```python
from build123d import *

# Parameters (mm, degrees)
SKETCH1_W           = 292.1
SKETCH1_H           = 158.75
BOSS_EXTRUDE1_DEPTH = 6.35
SKETCH2_R           = 3.175
CUT_EXTRUDE2_DEPTH  = 6.35
SKETCH4_R           = 2.54
SKETCH4_R_2         = 1.651
SKETCH4_R_3         = 2.667
SKETCH4_R_4         = 1.69999914
SKETCH4_R_5         = 2.0955
CUT_EXTRUDE5_DEPTH  = 333.512097524


with BuildPart() as part:
    # Sketch1 → Boss-Extrude1 (new body)
    with BuildSketch(Plane(origin=(0, 0, 0), x_dir=(1, 0, 0), z_dir=(0, 1, 0))):
        with Locations((146.05, 79.375)):
            Rectangle(SKETCH1_W, SKETCH1_H)
    extrude(amount=BOSS_EXTRUDE1_DEPTH)

    # Sketch2 → Cut-Extrude2 (cut)
    with BuildSketch(Plane(origin=(0, 6.35, 0), x_dir=(1, 0, 0), z_dir=(0, 1, 0))):
        with Locations(Location((146.05, 12.7, 0), (0, 0, 270))):
            Circle(SKETCH2_R)
        with Locations(Location((247.65, 12.7, 0), (0, 0, 270))):
            Circle(SKETCH2_R)
        with Locations(Location((44.45, 12.7, 0), (0, 0, 270))):
            Circle(SKETCH2_R)
    extrude(amount=-CUT_EXTRUDE2_DEPTH, mode=Mode.SUBTRACT)

    # Sketch4 → Cut-Extrude5 (cut, through all)
    with BuildSketch(Plane(origin=(0, 6.35, 0), x_dir=(1, 0, 0), z_dir=(0, 1, 0))):
        with Locations(Location((88.2015, 92.075, 0), (0, 0, 270))):
            Circle(SKETCH4_R)
        with Locations(Location((44.45, 111.125, 0), (0, 0, 270))):
            Circle(SKETCH4_R_2)
        with Locations(Location((44.45, 79.375, 0), (0, 0, 270))):
            Circle(SKETCH4_R_2)
        with Locations(Location((44.45, 47.625, 0), (0, 0, 270))):
            Circle(SKETCH4_R_2)
        with Locations(Location((10.795, 111.125, 0), (0, 0, 270))):
            Circle(SKETCH4_R_2)
        with Locations(Location((10.795, 79.375, 0), (0, 0, 270))):
            Circle(SKETCH4_R_2)
        with Locations(Location((10.795, 47.625, 0), (0, 0, 270))):
            Circle(SKETCH4_R_2)
        with Locations(Location((139.0015, 92.075, 0), (0, 0, 270))):
            Circle(SKETCH4_R)
        with Locations(Location((189.8015, 92.075, 0), (0, 0, 270))):
            Circle(SKETCH4_R)
        with Locations(Location((218.4146, 49.9364, 0), (0, 0, 270))):
            Circle(SKETCH4_R)
        with Locations(Location((285.0896, 49.9364, 0), (0, 0, 270))):
            Circle(SKETCH4_R)
        with Locations(Location((268.097, 139.3, 0), (0, 0, 270))):
            Circle(SKETCH4_R_3)
        with Locations(Location((268.097, 89.3, 0), (0, 0, 270))):
            Circle(SKETCH4_R_3)
        with Locations(Location((201.40419192, 147.125001204, 0), (0, 0, 270))):
            Circle(SKETCH4_R_4)
        with Locations(Location((157.90419256, 147.124999631, 0), (0, 0, 270))):
            Circle(SKETCH4_R_4)
        with Locations(Location((139.83529192, 147.125001204, 0), (0, 0, 270))):
            Circle(SKETCH4_R_4)
        with Locations(Location((96.33529256, 147.124999631, 0), (0, 0, 270))):
            Circle(SKETCH4_R_4)
        with Locations(Location((78.26639192, 147.125001204, 0), (0, 0, 270))):
            Circle(SKETCH4_R_4)
        with Locations(Location((34.76639256, 147.124999631, 0), (0, 0, 270))):
            Circle(SKETCH4_R_4)
        with Locations(Location((157.90419746, 11.624998851, 0), (0, 0, 270))):
            Circle(SKETCH4_R_4)
        with Locations(Location((201.40419682, 11.625000424, 0), (0, 0, 270))):
            Circle(SKETCH4_R_4)
        with Locations(Location((139.83529682, 11.625000424, 0), (0, 0, 270))):
            Circle(SKETCH4_R_4)
        with Locations(Location((96.33529746, 11.624998851, 0), (0, 0, 270))):
            Circle(SKETCH4_R_4)
        with Locations(Location((78.26639682, 11.625000424, 0), (0, 0, 270))):
            Circle(SKETCH4_R_4)
        with Locations(Location((34.76639746, 11.624998851, 0), (0, 0, 270))):
            Circle(SKETCH4_R_4)
        with Locations(Location((218.69969445, 141.2875, 0), (0, 0, 270))):
            Circle(SKETCH4_R_5)
        with BuildLine():
            Line((92.33531063, 130.175), (92.33531063, 120.65))
            ThreePointArc((92.33531063, 120.65), (89.16031063, 117.475), (85.98531063, 120.65))
            Line((85.98531063, 120.65), (85.98531063, 130.175))
            ThreePointArc((85.98531063, 130.175), (89.16031063, 133.35), (92.33531063, 130.175))
        make_face()
        with BuildLine():
            Line((30.76641063, 130.175), (30.76641063, 120.65))
            ThreePointArc((30.76641063, 120.65), (27.59141063, 117.475), (24.41641063, 120.65))
            Line((24.41641063, 120.65), (24.41641063, 130.175))
            ThreePointArc((24.41641063, 130.175), (27.59141063, 133.35), (30.76641063, 130.175))
        make_face()
        with BuildLine():
            Line((153.90421063, 130.175), (153.90421063, 120.65))
            ThreePointArc((153.90421063, 120.65), (150.72921063, 117.475), (147.55421063, 120.65))
            Line((147.55421063, 120.65), (147.55421063, 130.175))
            ThreePointArc((147.55421063, 130.175), (150.72921063, 133.35), (153.90421063, 130.175))
        make_face()
        with BuildLine():
            Line((153.90421063, 38.1), (153.90421063, 28.575))
            ThreePointArc((153.90421063, 28.575), (150.72921063, 25.4), (147.55421063, 28.575))
            Line((147.55421063, 28.575), (147.55421063, 38.1))
            ThreePointArc((147.55421063, 38.1), (150.72921063, 41.275), (153.90421063, 38.1))
        make_face()
        with BuildLine():
            Line((30.76641063, 38.1), (30.76641063, 28.575))
            ThreePointArc((30.76641063, 28.575), (27.59141063, 25.4), (24.41641063, 28.575))
            Line((24.41641063, 28.575), (24.41641063, 38.1))
            ThreePointArc((24.41641063, 38.1), (27.59141063, 41.275), (30.76641063, 38.1))
        make_face()
        with BuildLine():
            Line((92.33531063, 38.1), (92.33531063, 28.575))
            ThreePointArc((92.33531063, 28.575), (89.16031063, 25.4), (85.98531063, 28.575))
            Line((85.98531063, 28.575), (85.98531063, 38.1))
            ThreePointArc((85.98531063, 38.1), (89.16031063, 41.275), (92.33531063, 38.1))
        make_face()
        with BuildLine():
            Line((68.466400276, 149.625002844), (43.066400276, 149.625000636))
            ThreePointArc((43.066400276, 149.625000636), (40.821336067, 150.554938716), (39.8914, 152.800002844))
            Line((39.8914, 152.800002844), (39.8914, 158.75))
            Line((39.8914, 158.75), (71.6414, 158.75))
            Line((71.6414, 158.75), (71.6414, 152.800002844))
            ThreePointArc((71.6414, 152.800002844), (70.711464128, 150.554938912), (68.466400276, 149.625002844))
        make_face()
        with BuildLine():
            Line((101.4603, 152.800000636), (101.4603, 158.75))
            Line((101.4603, 158.75), (133.210297791, 158.75))
            Line((133.210297791, 158.75), (133.210297791, 152.800000636))
            ThreePointArc((133.210297791, 152.800000636), (132.280362566, 150.554938265), (130.035300276, 149.625002844))
            Line((130.035300276, 149.625002844), (104.635300276, 149.625000636))
            ThreePointArc((104.635300276, 149.625000636), (102.390236067, 150.554936508), (101.4603, 152.800000636))
        make_face()
        with BuildLine():
            Line((194.779197791, 158.75), (163.0292, 158.75))
            Line((163.0292, 158.75), (163.0292, 152.800000636))
            ThreePointArc((163.0292, 152.800000636), (163.959136067, 150.554936508), (166.204200276, 149.625000636))
            Line((166.204200276, 149.625000636), (191.604200276, 149.625002844))
            ThreePointArc((191.604200276, 149.625002844), (193.849262566, 150.554938265), (194.779197791, 152.800000636))
            Line((194.779197791, 152.800000636), (194.779197791, 158.75))
        make_face()
    extrude(amount=-CUT_EXTRUDE5_DEPTH, mode=Mode.SUBTRACT)


solid = part.part
```
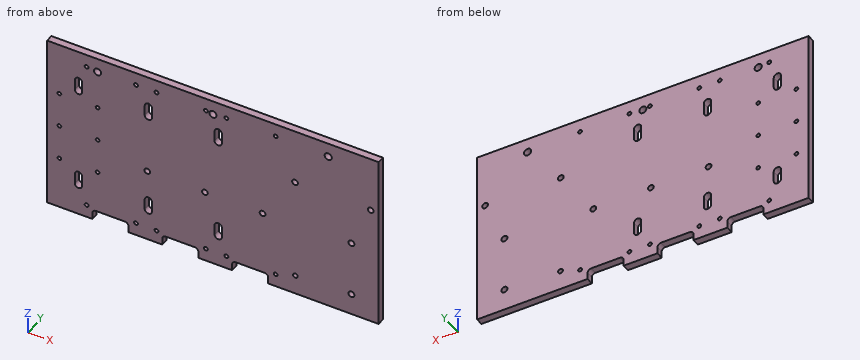
For this review, take the finished solid that the model builds, in its own axes (mm). Round coordinates to 2 decimals unless told otherwise and drop trailing zeros. Write each loop counter-clockwise with the first axis right and the second up, starting at its lowest first coordinate (ties: lowest second). Pieces come first, ordered by that corner, then holes. Notation, with made-up numbers: (89, -29.75) -> (123, -29.75) arc R28 ccw to (123, 8.25) -> close; hole circle Ø3 at (30, 18). An arc over 180 degrees is marked (long way). Use one line per item in the form item = value.
Q1. Consider section B-B (y = 1.75). State how many separate pieces and enclosed holes the cut face has, then the cut area to 3 significant figures.
Resolved:
separate_pieces = 1
enclosed_holes = 35
area = 44,500 mm²
Q2. To check wall thickness, follow probe 1 along X at (y, z) = (2, -29.5); probe 2 along X at (y, z) = (3.5, -133); probe 3 along Z at (x, y) = (87, 5). State the ranges of each line that lie inside material, in increasing order. Write a range as from..to.
Resolved:
probe_1 = 0..24.42, 30.77..85.99, 92.34..147.55, 153.9..292.1
probe_2 = 0..26.14, 29.04..87.71, 90.61..149.28, 152.18..292.1
probe_3 = -158.75..-132.5, -118.32..-94.31, -89.84..-40.43, -26.25..0
Q3. Consider section A-A (x = 247.65). State the section outline as (y, z) points (3 decimals).
Resolved:
outline = (0, -158.75) -> (6.35, -158.75) -> (6.35, -15.875) -> (0, -15.875) -> close; (0, -9.525) -> (6.35, -9.525) -> (6.35, 0) -> (0, 0) -> close
Q4. Clearance check with flat-ended pins moving along their axes: pin 1 Ø5.5 at (x, z) = (44.45, -111.125) entering from -Y; pin 2 Ø4 at (x, z) = (44.45, -12.7) entering from -Y. State where each tip first meets the part, or that it passes through.
Resolved:
pin_1 = 0
pin_2 = through
